The listing builds one solid part. Answer for the finished solid, in the listing's coordinates (mm). A direction names the side the tool comes from. Give positions to 0.01 mm unless a question says otherwise; leave off trailing zeros. Order: outer loops, then holes, each group sorted by start corner. A loop starts at its lowest first (then second) coordinate and runs counter-clockwise, first axis right, second up. Notation, with made-up numbers: (78.25, 8) - (137.25, 8) arc R28 ccw to (137.25, 31) - close; hole circle Ø5 at (5, 79). An arc over 180 degrees is marked (long way). Use CSV: the item, a comma, the result in double quotes.
```python
from build123d import *

# Parameters (mm, degrees)
SKETCH1_W             = 25
SKETCH1_H             = 61
SKETCH1_R             = 2
BOSS_EXTRUDE1_DEPTH   = 3
SKETCH1_W_2           = 20
BOSS_EXTRUDE1_2_DEPTH = 3
SKETCH3_W             = 5
SKETCH3_H             = 61
BOSS_EXTRUDE2_DEPTH   = 5
SKETCH4_W             = 5
SKETCH4_H             = 5
BOSS_EXTRUDE3_DEPTH   = 139
FILLET1_R             = 10
FILLET2_R             = 2


with BuildPart() as part:
    # Sketch1 → Boss-Extrude1 (new body)
    with BuildSketch(Plane(origin=(0, 0, 0), x_dir=(1, 0, 0), z_dir=(0, 1, 0))):
        with Locations((171.5, 30.5)):
            Rectangle(SKETCH1_W, SKETCH1_H)
        with Locations(Location((176.5, 10, 0), (0, 0, 90))):
            Circle(SKETCH1_R, mode=Mode.SUBTRACT)
        with Locations(Location((176.5, 51, 0), (0, 0, 270))):
            Circle(SKETCH1_R, mode=Mode.SUBTRACT)
    extrude(amount=BOSS_EXTRUDE1_DEPTH)



with BuildPart() as body_2:
    # Sketch1 → Boss-Extrude1 2 (new body)
    with BuildSketch(Plane(origin=(0, 0, 0), x_dir=(1, 0, 0), z_dir=(0, 1, 0))):
        with Locations((10, 30.5)):
            Rectangle(SKETCH1_W_2, SKETCH1_H)
        with Locations(Location((7.5, 10, 0), (0, 0, 270))):
            Circle(SKETCH1_R, mode=Mode.SUBTRACT)
        with Locations(Location((7.5, 51, 0), (0, 0, 90))):
            Circle(SKETCH1_R, mode=Mode.SUBTRACT)
    extrude(amount=BOSS_EXTRUDE1_2_DEPTH)


with BuildPart() as part_1:
    add(part.part)

    add(body_2.part)  # Boss-Extrude2 merges body 2
    # Sketch3 → Boss-Extrude2 (add)
    with BuildSketch(Plane(origin=(0, 3, 0), x_dir=(1, 0, 0), z_dir=(0, 1, 0))):
        with Locations((17.5, 30.5)):
            Rectangle(SKETCH3_W, SKETCH3_H)
        with Locations((161.5, 30.5)):
            Rectangle(SKETCH3_W, SKETCH3_H)
    extrude(amount=BOSS_EXTRUDE2_DEPTH)

    # Sketch4 → Boss-Extrude3 (add)
    with BuildSketch(Plane(origin=(20, 0, 0), x_dir=(0, 0, -1), z_dir=(1, 0, 0))):
        with Locations((2.5, 5.5)):
            Rectangle(SKETCH4_W, SKETCH4_H)
        with Locations((58.5, 5.5)):
            Rectangle(SKETCH4_W, SKETCH4_H)
    extrude(amount=BOSS_EXTRUDE3_DEPTH)

    # Fillet1
    fillet1_edges = [part_1.edges().sort_by_distance(p)[0] for p in [
        (184, 1.5, 0),
        (184, 1.5, -61),
        (0, 1.5, 0),
        (0, 1.5, -61),
    ]]
    fillet(fillet1_edges, radius=FILLET1_R)

    # Fillet2
    fillet2_edges = [part_1.edges().sort_by_distance(p)[0] for p in [
        (15, 3, -30.5),
        (15, 8, -30.5),
        (20, 3, -2.5),
        (20, 5.5, -5),
        (159, 3, -2.5),
        (159, 5.5, -5),
        (164, 3, -30.5),
        (164, 8, -30.5),
        (20, 5.5, -56),
        (20, 3, -58.5),
        (159, 3, -58.5),
        (159, 5.5, -56),
    ]]
    fillet(fillet2_edges, radius=FILLET2_R)


solid = part_1.part
```
Item 1: The part is cut by section C-C (x = 176.5). Give the vertices of the cut face in (y, z), and give its area (3 significant figures).
Taken from the geometry:
outline,"(0, -60.68) - (3, -60.68) - (3, -53) - (0, -53) - close; (0, -49) - (3, -49) - (3, -12) - (0, -12) - close; (0, -8) - (3, -8) - (3, -0.32) - (0, -0.32) - close"
area,"157 mm^2"
Item 2: Find the intervals of material crossed by line 1 along X through (y, z) = (1.1, -51); line 2 along X through (y, z) = (6.25, -7.5); line 3 along Z through (x, y) = (156, 3.75), in increasing order.
Taken from the geometry:
line 1,"0 to 5.5, 9.5 to 20, 159 to 174.5, 178.5 to 184"
line 2,"15.02 to 20, 159 to 163.98"
line 3,"-61 to -56, -5 to 0"
Item 3: The part is cut by section A-A (x = 146.5). Give the vertices of the cut face in (y, z), and give its area (3 significant figures).
Taken from the geometry:
outline,"(3, -61) - (8, -61) - (8, -56) - (3, -56) - close; (3, -5) - (8, -5) - (8, 0) - (3, 0) - close"
area,"50.0 mm^2"
Item 4: The mould has two halves that part along Z. Classify faces 6 (the face through (3.01, 1.52, -2.85)), 7 (the face through (0, 1, -30)), 8 (the face through (20, 4, -30)): +Z half, -Z half, draft (parallel to the pull), parting line (faces both ways), or undercut.
Taken from the geometry:
face 6,"+Z half"
face 7,"draft"
face 8,"undercut"
Item 5: The part is cut by section B-B (z = -30.5). Give the vertices of the cut face in (x, y), and give its area (3 significant figures).
Taken from the geometry:
outline,"(0, 0) - (20, 0) - (20, 8) - (17, 8) arc R2 ccw to (15, 6) - (15, 5) arc R2 cw to (13, 3) - (0, 3) - close; (159, 0) - (184, 0) - (184, 3) - (166, 3) arc R2 cw to (164, 5) - (164, 6) arc R2 ccw to (162, 8) - (159, 8) - close"
area,"185 mm^2"
Item 6: Each of these flat-tipped pins is pushed along its axis until it touches: pin 1 (0.8 mm diameter, centred on y = 5.5, z = -37, fed in from +X); pin 2 (14.5 mm diameter, centred on x = 6, z = -33.5, fed in from +Y); pin 3 (1.5 mm diameter, centred on x = 81, z = -3.5, fed in from -Y). Where does it stop, or does it pass through?
Taken from the geometry:
pin 1,"x = 164"
pin 2,"y = 3.02"
pin 3,"y = 3"
Item 7: Which of the six approach directions +Z, -Z, +X, -X, +Y, -Y give full straight-line access (tool end or side, diameter ignored) to faces 1 (the face through (6, 3, -31)), 2 (the face through (175, 3, -31)), 3 (the face through (78, 8, -57)), 4 (the face through (89, 5, -56)), 5 (the face through (89, 3, -58))?
Taken from the geometry:
face 1,"+Z, -Z, -X, +Y"
face 2,"+Z, -Z, +X, +Y"
face 3,"+Z, -Z, +X, -X, +Y"
face 4,"+Y, -Y"
face 5,"+Z, -Z, -Y"
